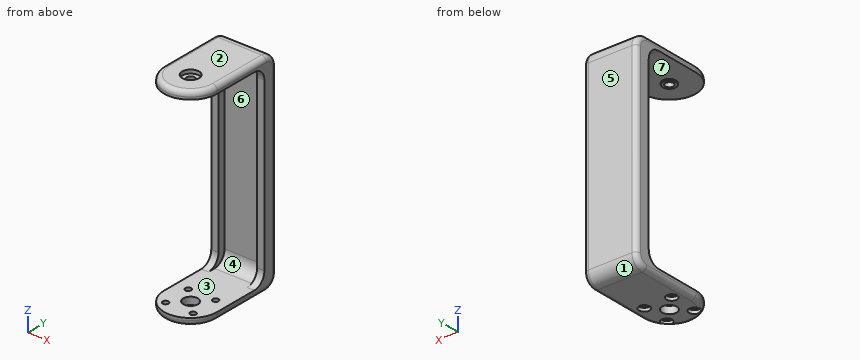
from build123d import *

# Parameters (mm, degrees)
ESBO_O1_R                                            = 3.05
RESSALTO_EXTRUS_O1_DEPTH                             = 3
ESBO_O2_W                                            = 22
ESBO_O2_H                                            = 82.35
RESSALTO_EXTRUS_O2_DEPTH                             = 3
RESSALTO_EXTRUS_O3_START                             = 3
RESSALTO_EXTRUS_O3_DEPTH                             = 3
ESBO_O6_W                                            = 85.35
ESBO_O6_H                                            = 6
RESSALTO_EXTRUS_O5_DEPTH                             = 3
ESBO_O7_R                                            = 2.75
RESSALTO_EXTRUS_O6_DEPTH                             = 0.6
REBAIXO_PARA_PARAFUSO_COM_CABE_A_PANELA_D            = 3.4
REBAIXO_PARA_PARAFUSO_COM_CABE_A_PANELA_CBORE_D      = 7
REBAIXO_PARA_PARAFUSO_COM_CABE_A_PANELA_CBORE_DEPTH  = 1.5
REBAIXO_PARA_PARAFUSO_COM_CABE_A_REDONDA_D           = 2.4
REBAIXO_PARA_PARAFUSO_COM_CABE_A_REDONDA_DEPTH       = 3
REBAIXO_PARA_PARAFUSO_COM_CABE_A_REDONDA_CBORE_D     = 4.4
REBAIXO_PARA_PARAFUSO_COM_CABE_A_REDONDA_CBORE_DEPTH = 1.4
PADR_OCIRCULAR1_COUNT                                = 4
FILETE1_R                                            = 5
FILETE2_R                                            = 5
FILETE3_R                                            = 2


with BuildPart() as part:
    # Esboço1 → Ressalto-extrusão1 (new body)
    with BuildSketch(Plane.XY):
        with BuildLine():
            Line((11, -1.428145739), (11, 25.071854261))
            Line((11, 25.071854261), (-11, 25.071854261))
            Line((-11, 25.071854261), (-11, -1.428145739))
            ThreePointArc((-11, -1.428145739), (0, -12.428145739), (11, -1.428145739))
        make_face()
        with Locations((0, -1.428145739)):
            Circle(ESBO_O1_R, mode=Mode.SUBTRACT)
    extrude(amount=-RESSALTO_EXTRUS_O1_DEPTH)

    # Esboço2 → Ressalto-extrusão2 (add)
    with BuildSketch(Plane(origin=(0, 25.071854261, 0), x_dir=(1, 0, 0), z_dir=(0, 1, 0))):
        with Locations((0, -38.175)):
            Rectangle(ESBO_O2_W, ESBO_O2_H)
    extrude(amount=RESSALTO_EXTRUS_O2_DEPTH)

    # Esboço3 → Ressalto-extrusão3 (add)
    with BuildSketch(Plane.XY.offset(79.35).offset(RESSALTO_EXTRUS_O3_START)):
        with BuildLine():
            Line((11, 28.071854261), (-11, 28.071854261))
            Line((-11, 28.071854261), (-11, -1.428145739))
            ThreePointArc((-11, -1.428145739), (0, -12.428145739), (11, -1.428145739))
            Line((11, -1.428145739), (11, 28.071854261))
        make_face()
    extrude(amount=-RESSALTO_EXTRUS_O3_DEPTH)

    # Esboço6 → Ressalto-extrusão5 (add)
    with BuildSketch(Plane(origin=(11, 0, 0), x_dir=(0, 0, -1), z_dir=(1, 0, 0))):
        with Locations((-39.675, 25.071854261)):
            Rectangle(ESBO_O6_W, ESBO_O6_H)
    ressalto_extrus_o5 = extrude(amount=-RESSALTO_EXTRUS_O5_DEPTH)

    # Espelhar1: Ressalto-extrusão5 across plane
    add(ressalto_extrus_o5.mirror(Plane(origin=(0, 0, 0), x_dir=(0, 0, 1), z_dir=(1, 0, 0))))

    # Esboço7 → Ressalto-extrusão6 (add)
    with BuildSketch(Plane(origin=(0, 0, 79.35), x_dir=(-1, 0, 0), z_dir=(0, 0, -1))):
        with Locations(Location((0, -1.428145739, 0), (0, 0, 180))):
            Circle(ESBO_O7_R)
    extrude(amount=RESSALTO_EXTRUS_O6_DEPTH)

    # Rebaixo para parafuso com cabeça panela de M31 (through all)
    with Locations(Plane.XY.offset(82.35)):
        with Locations((0, -1.428145739)):
            CounterBoreHole(REBAIXO_PARA_PARAFUSO_COM_CABE_A_PANELA_D / 2, REBAIXO_PARA_PARAFUSO_COM_CABE_A_PANELA_CBORE_D / 2, REBAIXO_PARA_PARAFUSO_COM_CABE_A_PANELA_CBORE_DEPTH)

    # Rebaixo para parafuso com cabeça redonda de M21
    with Locations(Plane(origin=(0, 0, -3), x_dir=(-1, 0, 0), z_dir=(0, 0, -1))):
        with Locations((-5.624741587, 4.260639903)):
            rebaixo_para_parafuso_com_cabe_a_redonda = CounterBoreHole(REBAIXO_PARA_PARAFUSO_COM_CABE_A_REDONDA_D / 2, REBAIXO_PARA_PARAFUSO_COM_CABE_A_REDONDA_CBORE_D / 2, REBAIXO_PARA_PARAFUSO_COM_CABE_A_REDONDA_CBORE_DEPTH, depth=REBAIXO_PARA_PARAFUSO_COM_CABE_A_REDONDA_DEPTH)

    # PadrãoCircular1: Rebaixo para parafuso com cabeça redonda de M21 ×4 about axis
    padr_ocircular1_axis = Axis((0, -1.428145739, 0), (0, 0, 1))
    for i in range(1, PADR_OCIRCULAR1_COUNT):
        add(rebaixo_para_parafuso_com_cabe_a_redonda.rotate(padr_ocircular1_axis, i * 360 / PADR_OCIRCULAR1_COUNT), mode=Mode.SUBTRACT)

    # Filete1
    filete1_edges = [part.edges().sort_by_distance(p)[0] for p in [
        (0, 25.071854261, 0),
        (0, 25.071854261, 79.35),
        (0, 28.071854261, -3),
        (0, 28.071854261, 82.35),
    ]]
    fillet(filete1_edges, radius=FILETE1_R)

    # Filete2
    # the kernel refuses this fillet: 5 mm, written as the material it adds along each edge
    with BuildSketch(Plane(origin=(11, 22.071854261, 0.417424305), x_dir=(0, -0.9965332502141475, -0.0831954398848114), z_dir=(-1, 0, 0)), Plane(origin=(-11, 22.071854261, 78.932575695), x_dir=(0, -0.9965332502141476, 0.0831954398848087), z_dir=(1, 0, 0))) as filete2_piece_1:
        with BuildLine():
            CenterArc((4.60141685, 4.982666251), FILETE2_R, 184.772263604, 90)
            Line((-0.381249401, 4.566689052), (-0.879516026, 4.525091332))
            Line((-0.879516026, 4.525091332), (-0.498266625, -0.04159772))
            Line((-0.498266625, -0.04159772), (-0.16118171, -0.473307993))
            ThreePointArc((-0.16118171, -0.473307993), (2.069392019, -0.747852945), (5.05899177, -0.498266625))
            Line((5.05899177, -0.498266625), (5.01739405, 0))
        make_face()
    extrude(amount=3)
    with BuildSketch(Plane(origin=(-11, 22.071854261, 0.417424305), x_dir=(0, -0.9965332502141475, -0.08319543988481146), z_dir=(1, 0, 0))) as filete2_piece_2:
        with BuildLine():
            CenterArc((4.60141685, -4.982666251), FILETE2_R, 85.227736396, 90)
            Line((-0.381249401, -4.566689052), (-0.879516026, -4.525091332))
            Line((-0.879516026, -4.525091332), (-0.498266625, 0.04159772))
            Line((-0.498266625, 0.04159772), (-0.16118171, 0.473307993))
            ThreePointArc((-0.16118171, 0.473307993), (2.069392019, 0.747852945), (5.05899177, 0.498266625))
            Line((5.05899177, 0.498266625), (5.01739405, 0))
        make_face()
    extrude(amount=3)
    with BuildSketch(Plane(origin=(11, 22.071854261, 78.932575695), x_dir=(0, 0, -1), z_dir=(-1, 0, 0))) as filete2_piece_3:
        with BuildLine():
            CenterArc((4.582575695, 5), FILETE2_R, 180, 90)
            Line((-0.417424305, 5), (-0.917424305, 5))
            ThreePointArc((-0.917424305, 5), (-0.917424305, 2), (-0.458257569, -0.2))
            Line((-0.458257569, -0.2), (0, -0.5))
            Line((0, -0.5), (4.582575695, -0.5))
            Line((4.582575695, -0.5), (4.582575695, 0))
        make_face()
    extrude(amount=3)

    # Filete3
    # the kernel refuses this fillet: 2 mm, written as the material it takes off along each edge
    with BuildSketch(Plane(origin=(-11, 28.071854261, 2), x_dir=(1, 0, 0), z_dir=(0, 0, 1))) as filete3_piece_1:
        with BuildLine():
            CenterArc((FILETE3_R, -FILETE3_R), FILETE3_R, 90, 90)
            Line((0, -FILETE3_R), (0, 0))
            Line((0, 0), (FILETE3_R, 0))
        make_face()
    extrude(amount=75.35, mode=Mode.SUBTRACT)
    with BuildSketch(Plane(origin=(11, 28.071854261, 2), x_dir=(-1, 0, 0), z_dir=(0, 0, 1))) as filete3_piece_2:
        with BuildLine():
            CenterArc((FILETE3_R, FILETE3_R), FILETE3_R, 180, 90)
            Line((0, FILETE3_R), (0, 0))
            Line((0, 0), (FILETE3_R, 0))
        make_face()
    extrude(amount=75.35, mode=Mode.SUBTRACT)
    with BuildSketch(Plane(origin=(-11, -1.428145739, -3), x_dir=(1, 0, 0), z_dir=(0, 1, 0)), Plane(origin=(-11, 23.071854261, 82.35), x_dir=(1, 0, 0), z_dir=(0, -1, 0))) as filete3_piece_3:
        with BuildLine():
            CenterArc((FILETE3_R, -FILETE3_R), FILETE3_R, 90, 90)
            Line((0, -FILETE3_R), (0, 0))
            Line((0, 0), (FILETE3_R, 0))
        make_face()
    extrude(amount=24.5, mode=Mode.SUBTRACT)
    with BuildSketch(Plane(origin=(-11, 23.071854261, 77.35), x_dir=(0, 1, 0), z_dir=(0, 0, -1))) as filete3_piece_4:
        with BuildLine():
            CenterArc((5 - FILETE3_R, FILETE3_R), FILETE3_R, 270, 90)
            Line((5 - FILETE3_R, 0), (5, 0))
            Line((5, 0), (5, FILETE3_R))
        make_face()
    revolve(axis=Axis((-11, 23.071854261, 77.35), (1, 0, 0)), revolution_arc=90, mode=Mode.SUBTRACT)
    with BuildSketch(Plane(origin=(-11, 23.071854261, 2), x_dir=(0, 0, -1), z_dir=(0, -1, 0))) as filete3_piece_5:
        with BuildLine():
            CenterArc((5 - FILETE3_R, FILETE3_R), FILETE3_R, 270, 90)
            Line((5 - FILETE3_R, 0), (5, 0))
            Line((5, 0), (5, FILETE3_R))
        make_face()
    revolve(axis=Axis((-11, 23.071854261, 2), (1, 0, 0)), revolution_arc=90, mode=Mode.SUBTRACT)
    with BuildSketch(Plane(origin=(11, 23.071854261, 77.35), x_dir=(0, 1, 0), z_dir=(0, 0, -1))) as filete3_piece_6:
        with BuildLine():
            CenterArc((5 - FILETE3_R, -FILETE3_R), FILETE3_R, 0, 90)
            Line((5 - FILETE3_R, 0), (5, 0))
            Line((5, 0), (5, -FILETE3_R))
        make_face()
    revolve(axis=Axis((11, 23.071854261, 77.35), (1, 0, 0)), revolution_arc=90, mode=Mode.SUBTRACT)
    with BuildSketch(Plane(origin=(11, 23.071854261, 2), x_dir=(0, 0, -1), z_dir=(0, -1, 0))) as filete3_piece_7:
        with BuildLine():
            CenterArc((5 - FILETE3_R, -FILETE3_R), FILETE3_R, 0, 90)
            Line((5 - FILETE3_R, 0), (5, 0))
            Line((5, 0), (5, -FILETE3_R))
        make_face()
    revolve(axis=Axis((11, 23.071854261, 2), (1, 0, 0)), revolution_arc=90, mode=Mode.SUBTRACT)
    with BuildSketch(Plane(origin=(11, 23.071854261, 82.35), x_dir=(-1, 0, 0), z_dir=(0, -1, 0)), Plane(origin=(11, -1.428145739, -3), x_dir=(-1, 0, 0), z_dir=(0, 1, 0))) as filete3_piece_8:
        with BuildLine():
            CenterArc((FILETE3_R, FILETE3_R), FILETE3_R, 180, 90)
            Line((0, FILETE3_R), (0, 0))
            Line((0, 0), (FILETE3_R, 0))
        make_face()
    extrude(amount=24.5, mode=Mode.SUBTRACT)
    with BuildSketch(Plane(origin=(0, -1.428145739, 82.35), x_dir=(-1, 0, 0), z_dir=(0, 1, 0))) as filete3_piece_9:
        with BuildLine():
            CenterArc((11 - FILETE3_R, -FILETE3_R), FILETE3_R, 0, 90)
            Line((11, -FILETE3_R), (11, 0))
            Line((11, 0), (11 - FILETE3_R, 0))
        make_face()
    revolve(axis=Axis((0, -1.428145739, 82.35), (0, 0, 1)), revolution_arc=180, mode=Mode.SUBTRACT)
    with BuildSketch(Plane(origin=(0, -1.428145739, -3), x_dir=(-1, 0, 0), z_dir=(0, 1, 0))) as filete3_piece_10:
        with BuildLine():
            CenterArc((11 - FILETE3_R, FILETE3_R), FILETE3_R, 270, 90)
            Line((11, FILETE3_R), (11, 0))
            Line((11, 0), (11 - FILETE3_R, 0))
        make_face()
    revolve(axis=Axis((0, -1.428145739, -3), (0, 0, 1)), revolution_arc=180, mode=Mode.SUBTRACT)


solid = part.part
Verification items for the finished model (mm, model axes). Face numbers are marked on the shaded views. A direction names the side the tool comes from. Give positions to 0.01 mm unless a question says otherwise; leave off trailing zeros. Loops run counter-clockwise (first coordinate to the right, second up) from the corner with the lowest first, then second, coordinate; pieces in that order, holes last.
1. Cross-section at B-B on x = 0. Count the separate pieces of the cut face and the enclosed holes in it, and give its area (3 significant figures).
Derived:
separate pieces: 3
enclosed holes: 0
area: 447 mm2
2. Cross-section at C-C on z = 54. Record the cut outline in (x, y).
Derived:
outline: (-11, 22.07) - (-8, 22.07) - (-8, 25.07) - (8, 25.07) - (8, 22.07) - (11, 22.07) - (11, 26.07) arc R2 ccw to (9, 28.07) - (-9, 28.07) arc R2 ccw to (-11, 26.07) - close
3. Release check for a two-part mould opening along Z. For the marked faces 1, 2, 3 and 4 record: +Z half, -Z half, draft (parallel to the pull), parting line (faces both ways), or undercut.
Derived:
face 1: -Z half
face 2: +Z half
face 3: undercut
face 4: undercut
4. Cross-section at A-A on y = 7.5. Record the cut outline in (x, z).
Derived:
outline: (-11, -1) arc R2 ccw to (-9, -3) - (9, -3) arc R2 ccw to (11, -1) - (11, 0) - (-11, 0) - close; (-11, 79.35) - (11, 79.35) - (11, 80.35) arc R2 ccw to (9, 82.35) - (-9, 82.35) arc R2 ccw to (-11, 80.35) - close
5. Tool access check on the marked faces 5, 6 and 7. Record the directions out of +Z, -Z, +X, -X, +Y, -Y that give a thin tool (end or side, any length) a straight path to the whole face; none if there is none.
Derived:
face 5: +Z, -Z, +X, -X, +Y
face 6: -Y
face 7: none
6. Cross-section at D-D on y = 21. Record the cut outline in (x, z), and give its area (3 significant figures).
Derived:
outline: (-11, -1) arc R2 ccw to (-9, -3) - (9, -3) arc R2 ccw to (11, -1) - (11, 1.91) - (8, 1.91) - (8, 0.09) - (-8, 0.09) - (-8, 1.91) - (-11, 1.91) - close; (-11, 77.44) - (-8, 77.44) - (-8, 79.26) - (8, 79.26) - (8, 77.44) - (11, 77.44) - (11, 80.35) arc R2 ccw to (9, 82.35) - (-9, 82.35) arc R2 ccw to (-11, 80.35) - close
area: 154 mm2
7. Go/stop test with flat-tipped pins: P1, Ø1.3, axis at x = 6, y = -8, coming from the -Z side; P2, Ø2.5, axis at x = -9, z = 40, coming from the -Y side; P3, Ø12, axis at y = 15.5, z = 22.5, coming from the +X side; P4, Ø1.5, axis at x = -2.5, z = 36.5, coming from the -Y side. Record where each tip stops, or that it passes through.
Derived:
P1: stops at z = -1.6
P2: stops at y = 22.07
P3: passes through
P4: stops at y = 25.07
8. Material ranges on probe 1 along Z at (x, y) = (-5.25, 6); probe 2 along X at (y, z) = (22.5, 74.5); probe 3 along Z at (x, y) = (-6, 12), recorded low to high.
Derived:
probe 1: z = -1.6 to 0, 79.35 to 82.35
probe 2: x = -11 to -8, 8 to 11
probe 3: z = -3 to 0, 79.35 to 82.35
